Could you check a few things on this model? Use its own coordinates, in mm. A direction names the side the tool comes from. Coordinates: 2 decimals unless noted, no trailing zeros. Loops run counter-clockwise (first coordinate to the right, second up) from the corner with the lowest first, then second, coordinate; pieces in that order, holes last.
from build123d import *

# Parameters (mm, degrees)
F1_DEPTH = 25
F2_COUNT = 12
F5_D     = 4
F6_R     = 40
F7_DEPTH = 25.001


with BuildPart() as f1:
    # F0 (on Top) → F1 (new body)
    with BuildSketch(Plane.XY):
        with BuildLine():
            ThreePointArc((-4.9937460889, 49.75), (-33.5433502766, -37.0788841825), (50, 0))
            ThreePointArc((50, 0), (37.0788841825, 33.5433502766), (4.9937460889, 49.75))
            ThreePointArc((4.9937460889, 49.75), (0, 45), (-4.9937460889, 49.75))
        make_face()
        with BuildLine():
            ThreePointArc((-4.9937460889, 49.75), (0, 45), (4.9937460889, 49.75))
            ThreePointArc((4.9937460889, 49.75), (0, 50), (-4.9937460889, 49.75))
        make_face()
        with BuildLine():
            ThreePointArc((-4.9937460889, 49.75), (0, 50), (4.9937460889, 49.75))
            ThreePointArc((4.9937460889, 49.75), (4.9984362777, 49.8749608947), (5, 50))
            ThreePointArc((5, 50), (-0.1250391053, 54.9984362777), (-4.9937460889, 49.75))
        make_face()
    extrude(amount=F1_DEPTH)


with BuildPart() as f2_1:
    # F2: instance of F1
    add(f1.part.rotate(Axis((0, 0, 0), (0, 0, -1)), 1 * 360 / F2_COUNT))


with BuildPart() as f2_2:
    # F2: instance of F1
    add(f1.part.rotate(Axis((0, 0, 0), (0, 0, -1)), 2 * 360 / F2_COUNT))


with BuildPart() as f2_3:
    # F2: instance of F1
    add(f1.part.rotate(Axis((0, 0, 0), (0, 0, -1)), 3 * 360 / F2_COUNT))


with BuildPart() as f2_4:
    # F2: instance of F1
    add(f1.part.rotate(Axis((0, 0, 0), (0, 0, -1)), 4 * 360 / F2_COUNT))


with BuildPart() as f2_5:
    # F2: instance of F1
    add(f1.part.rotate(Axis((0, 0, 0), (0, 0, -1)), 5 * 360 / F2_COUNT))


with BuildPart() as f2_6:
    # F2: instance of F1
    add(f1.part.rotate(Axis((0, 0, 0), (0, 0, -1)), 6 * 360 / F2_COUNT))


with BuildPart() as f2_7:
    # F2: instance of F1
    add(f1.part.rotate(Axis((0, 0, 0), (0, 0, -1)), 7 * 360 / F2_COUNT))


with BuildPart() as f2_8:
    # F2: instance of F1
    add(f1.part.rotate(Axis((0, 0, 0), (0, 0, -1)), 8 * 360 / F2_COUNT))


with BuildPart() as f2_9:
    # F2: instance of F1
    add(f1.part.rotate(Axis((0, 0, 0), (0, 0, -1)), 9 * 360 / F2_COUNT))


with BuildPart() as f2_10:
    # F2: instance of F1
    add(f1.part.rotate(Axis((0, 0, 0), (0, 0, -1)), 10 * 360 / F2_COUNT))


with BuildPart() as f2_11:
    # F2: instance of F1
    add(f1.part.rotate(Axis((0, 0, 0), (0, 0, -1)), 11 * 360 / F2_COUNT))


with BuildPart() as f1_1:
    add(f1.part)

    # F3: union F2_5, F2_6, F2_1, F2_2, F2_3, F2_4, F2_11, F2_10, F2_7, F2_8, F2_9
    add(f2_5.part)
    add(f2_6.part)
    add(f2_1.part)
    add(f2_2.part)
    add(f2_3.part)
    add(f2_4.part)
    add(f2_11.part)
    add(f2_10.part)
    add(f2_7.part)
    add(f2_8.part)
    add(f2_9.part)

    # F5 (through all)
    with Locations(Plane(origin=(0, 0, 0), x_dir=(1, 0, 0), z_dir=(0, 0, -1))):
        with Locations((43.3012701892, -25), (25, -43.3012701892), (0, -49.75), (-25, -43.3012701892), (-43.3012701892, -25), (-50, 0), (-43.3012701892, 25), (-25, 43.3012701892), (0, 49.75), (25, 43.3012701892), (43.3012701892, 25), (49.75, 0)):
            Hole(F5_D / 2)

    # F6 (on face) → F7 (cut, through all)
    with BuildSketch(Plane(origin=(0, 0, 0), x_dir=(1, 0, 0), z_dir=(0, 0, -1))):
        Circle(F6_R)
    extrude(amount=-F7_DEPTH, mode=Mode.SUBTRACT)


solid = f1_1.part
1) Imagine slicing it at A-A on y = 0. List the corners of the cut face in (x, z) for me, plus the area to 3 significant figures.
2) Imagine slicing it at D-D on z = 8. State how many separate pieces and enclosed holes the cut face has, plus the area to 3 significant figures.
3) For faces 1 (the cylindrical face through (-48.325, -12.832, 12.325)), 2 (the cylindrical face through (13.05, 48.267, 12.325)), 3 (the cylindrical face through (-8.67, 39.05, 12.32)), 4 (the cylindrical face through (12.832, -48.325, 12.325)), which set-ups out of +Z, -Z, +X, -X, +Y, -Y let a thin tool reach every point of the face, with its end or its side?
4) If I drill on L1, parallel to Y at x = 0, z = 5.5; L2, parallel to X at y = 50, z = 15.25; L3, parallel to X at y = -42, z = 10.5, over which ranges is the centre line in solid material (lowest first)?
5) We'd pull the mould along X, two halves only. Please class faces 5 (the cylindrical face through (48.267, -13.05, 12.325)), 6 (the cylindrical face through (-48.267, 13.05, 12.325)), 7 (the cylindrical face through (-13.05, -48.267, 12.325)): released by +X, released by -X, zero draft, split by the parting line, or undercut.
6) Imagine slicing it at C-C on y = -37.5. List the corners of the cut face in (x, z) for me.
7) Will these pins go through, and if not, where does the flat tip stop? pin 1 (3 mm diameter, centred on x = 43.3, y = -25, fed in from +Z); pin 2 (10 mm diameter, centred on y = -40.5, z = 12, fed in from +X); pin 3 (3 mm diameter, centred on y = -37, z = 9.5, fed in from -X); pin 4 (3 mm diameter, centred on y = -29, z = 17, fed in from -X).
8) Imagine slicing it at B-B on x = -6.5. List the corners of the cut face in (y, z) for me, plus the area to 3 significant figures.
Solved:
1. outline: (-55, 0) - (-52, 0) - (-52, 25) - (-55, 25) - close; (-48, 0) - (-40, 0) - (-40, 25) - (-48, 25) - close; (40, 0) - (47.75, 0) - (47.75, 25) - (40, 25) - close; (51.75, 0) - (55, 0) - (55, 25) - (51.75, 25) - close
1. area: 550 mm2
2. separate pieces: 1
2. enclosed holes: 13
2. area: 3,160 mm2
3. face 1: +Z, -Z, -X
3. face 2: +Z, -Z, +Y
3. face 3: +Z, -Z
3. face 4: +Z, -Z, -Y
4. L1: y = -55 to -51.75, -47.75 to -40, 40 to 47.75, 51.75 to 55
4. L2: x = -5 to -1.98, 1.98 to 5
4. L3: x = -29.83 to -26.52, -23.48 to 23.48, 26.52 to 29.83
5. face 5: released by +X
5. face 6: released by -X
5. face 7: undercut
6. outline: (-33.07, 0) - (-13.92, 0) - (-13.92, 25) - (-33.07, 25) - close; (13.92, 0) - (33.07, 0) - (33.07, 25) - (13.92, 25) - close
7. pin 1: passes through
7. pin 2: stops at x = 35.21
7. pin 3: stops at x = -35.21
7. pin 4: stops at x = -47.63
8. outline: (-49.58, 0) - (-39.47, 0) - (-39.47, 25) - (-49.58, 25) - close; (39.47, 0) - (49.58, 0) - (49.58, 25) - (39.47, 25) - close
8. area: 505 mm2
